Work out the finished part from the listing and answer in its coordinate system (mm). Give positions to 0.01 mm unless a question says otherwise; leave off trailing zeros. Loops run counter-clockwise (first coordinate to the right, second up) from the corner with the lowest first, then second, coordinate; pieces in that order, holes last. Notation, with made-up numbers: M -18,-20.5 L 9,-20.5 A13 cw 9,-12.5 Z; hole C 88,-1.5 d2. An arc over 180 degrees is marked long. Use a Markdown table: item, result.
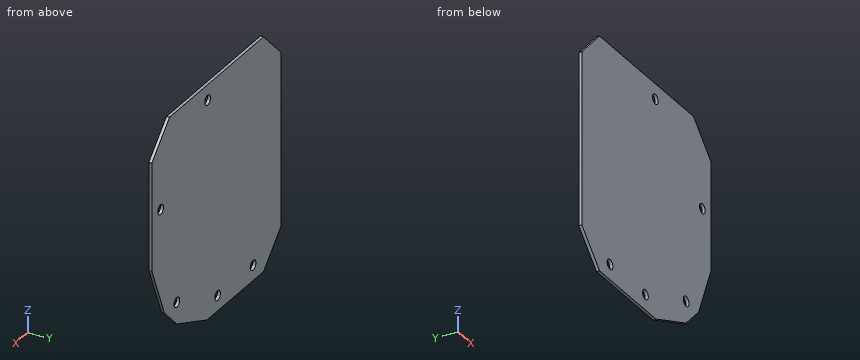
```python
from build123d import *

# Parameters (mm, degrees)
EXTRUDE_1_DEPTH     = 1
SKETCH_2_W          = 31.819805153
SKETCH_2_H          = 31.819805153
CUT_EXTRUDE_1_DEPTH = 10
CHAMFER_1_SIZE      = 10
SKETCH_4_R          = 1.6
CUT_EXTRUDE_3_DEPTH = 10
SKETCH_5_W          = 20
SKETCH_5_H          = 76.213203436
EXTRUDE_2_DEPTH     = 1
CHAMFER_2_SIZE      = 10
SKETCH_6_R          = 1.6
CUT_EXTRUDE_4_DEPTH = 10


with BuildPart() as part:
    # 草图1 → 凸台-拉伸1 (new body)
    with BuildSketch(Plane(origin=(0, 0, 0), x_dir=(1, 0, 0), z_dir=(0, 1, 0))):
        Polygon((0, 0), (53.033008589, 0), (53.033008589, 55), (0, 108.033008589), align=None)
    extrude(amount=EXTRUDE_1_DEPTH)

    # 草图2 → 切除-拉伸1 (cut)
    with BuildSketch(Plane.XZ):
        with Locations((15.909902577, -92.123106013)):
            Rectangle(SKETCH_2_W, SKETCH_2_H)
    extrude(amount=-CUT_EXTRUDE_1_DEPTH, mode=Mode.SUBTRACT)

    # 倒角1
    chamfer_1_edges = [part.edges().sort_by_distance(p)[0] for p in [
        (31.819805153, 0.5, -76.213203436),
        (53.033008589, 0.5, -55),
        (53.033008589, 0.5, 0),
    ]]
    chamfer(chamfer_1_edges, length=CHAMFER_1_SIZE)

    # 草图4 → 切除-拉伸3 (cut)
    with BuildSketch(Plane(origin=(0, 1, 0), x_dir=(1, 0, 0), z_dir=(0, 1, 0))):
        with Locations(Location((38.890872965, 62.071067812, 0), (0, 0, 270))):
            Circle(SKETCH_4_R)
        with Locations(Location((48.033008589, 27.5, 0), (0, 0, 270))):
            Circle(SKETCH_4_R)
        with Locations(Location((21.516504294, 5, 0), (0, 0, 270))):
            Circle(SKETCH_4_R)
    extrude(amount=-CUT_EXTRUDE_3_DEPTH, mode=Mode.SUBTRACT)

    # 草图5 → 凸台-拉伸2 (add)
    with BuildSketch(Plane.XZ):
        with Locations((-10, -38.106601718)):
            Rectangle(SKETCH_5_W, SKETCH_5_H)
    extrude(amount=-EXTRUDE_2_DEPTH)

    # 倒角2
    chamfer_2_edges = [part.edges().sort_by_distance(p)[0] for p in [
        (-20, 0.5, 0),
        (-20, 0.5, -76.213203436),
    ]]
    chamfer(chamfer_2_edges, length=CHAMFER_2_SIZE)

    # 草图6 → 切除-拉伸4 (cut)
    with BuildSketch(Plane.XZ):
        with Locations(Location((15.909902577, -71.213203436, 0), (0, 0, 270))):
            Circle(SKETCH_6_R)
        with Locations(Location((-4.090097423, -71.213203436, 0), (0, 0, 270))):
            Circle(SKETCH_6_R)
    extrude(amount=-CUT_EXTRUDE_4_DEPTH, mode=Mode.SUBTRACT)


solid = part.part
```
(1) A cutting plane is placed at B-B (y = 0.8). Write down the section's boundary in (x, z).
Entries:
| item | result |
|---|---|
| outline | M -20,-66.21 L -10,-76.21 L 21.82,-76.21 L 38.89,-69.14 L 45.96,-62.07 L 53.03,-45 L 53.03,-10 L 43.03,0 L -10,0 L -20,-10 Z; hole C -4.09,-71.21 d3.2; hole C 15.91,-71.21 d3.2; hole C 21.52,-5 d3.2; hole C 38.89,-62.07 d3.2; hole C 48.03,-27.5 d3.2 |
(2) Consider probe 1 along X at (y, z) = (0.85, -27.5); probe 2 along X at (y, z) = (0.45, -72); probe 3 along X at (y, z) = (0.5, -71). Determine where each line is inside the solid, lowest interval first. Write a range as [from, to].
Entries:
| item | result |
|---|---|
| probe 1 | x = [-20, 46.43], [49.63, 53.03] |
| probe 2 | x = [-14.21, -5.48], [-2.7, 14.52], [17.3, 31.99] |
| probe 3 | x = [-15.21, -5.68], [-2.5, 14.32], [17.5, 34.41] |
(3) Given P1, Ø2.5, axis at x = 48.03, z = -27.5, coming from the -Y side, flat-ended and moving along its own axis, determine where the tip first touches the part or whether it passes through.
Entries:
| item | result |
|---|---|
| P1 | passes through |
(4) A cutting plane is placed at A-A (z = -27.5). Write down the section's boundary in (x, y), and give its area (3 significant figures).
Entries:
| item | result |
|---|---|
| outline | M -20,0 L 46.43,0 L 46.43,1 L -20,1 Z; M 49.63,0 L 53.03,0 L 53.03,1 L 49.63,1 Z |
| area | 69.8 mm² |
(5) A cutting plane is placed at D-D (x = -14). Write down the section's boundary in (y, z).
Entries:
| item | result |
|---|---|
| outline | M 0,-72.21 L 1,-72.21 L 1,-4 L 0,-4 Z |
(6) A cutting plane is placed at C-C (z = -5). Write down the section's boundary in (x, y), and give its area (3 significant figures).
Entries:
| item | result |
|---|---|
| outline | M -15,0 L 19.92,0 L 19.92,1 L -15,1 Z; M 23.12,0 L 48.03,0 L 48.03,1 L 23.12,1 Z |
| area | 59.8 mm² |
